Design review of the part built by this model. Coordinates are the model's own, in mm. A direction names the side the tool comes from. Give positions to 0.01 mm unless a question says otherwise; leave off trailing zeros. Loops run counter-clockwise (first coordinate to the right, second up) from the corner with the lowest first, then second, coordinate; pieces in that order, holes last. Notation, with made-up numbers: M 84.5,15.25 L 120.5,15.25 A13 ccw 120.5,35.25 Z; hole C 51,34.5 d3. An arc over 180 degrees is marked long. Use a Markdown table: item, result. Add a question column.
(1) Draft analysis for pull direction X (two halves, no side actions). For faces 3 (the face through (-427, 7, -650)), 4 (the face through (-311.84, 8.526, -537.131)), 5 (the face through (-650, 7, -427)), 6 (the face through (-536.16, 8.526, -310.869)), state which applies: pulls with the +X half, pulls with the -X half, needs draft (parallel to the pull), parting line crosses it, or undercut.
(2) For faces 1 (the face through (-536.16, 8.526, -537.131)), 2 (the face through (-427, 14.5, -421)), list the 3-axis set-ups (+Z, -Z, +X, -X, +Y, -Y) from which the entire face can be reached by the end or side of a thin tool; tool diameter is ignored.
(3) Add section A-A, the plane x = -546. Give the boundary of the cut face in (y, z) (3 decimals), then the cut area to 3 significant figures.
(4) Insertion check: pin 1 Ø3.5 at (x, z) = (-281, -326) entering from -Y. The pin has a flat end and moves straight along its axis. Give the tip position at first contact, or say it passes through.
(5) For probe 1 along X at (y, z) = (9, -552); probe 2 along Z at (x, y) = (-567, 6); probe 3 along Z at (x, y) = (-515, 9), list the stretches that pass through material, from the lowest coordinate up.
```python
from build123d import *

# Parameters (mm, degrees)
SKETCH1_W               = 452
SKETCH1_H               = 452
BOSS_EXTRUDE1_DEPTH     = 15
SKETCH15_R              = 5.975
CUT_EXTRUDE12_DEPTH     = 120
MIRROR2_COPY_1_SKETCH_R = 5.975
MIRROR2_COPY_1_DEPTH    = 120
SKETCH16_R              = 3
CUT_EXTRUDE13_DEPTH     = 120
SKETCH17_R              = 4.1
SKETCH17_R_2            = 4.25
CUT_EXTRUDE14_DEPTH     = 120
MIRROR4_COPY_1_SKETCH_R = 3
MIRROR4_COPY_1_DEPTH    = 120


with BuildPart() as part:
    # Sketch1 → Boss-Extrude1 (new body)
    with BuildSketch(Plane.XZ.offset(0.5)):
        with Locations((-424, -424)):
            Rectangle(SKETCH1_W, SKETCH1_H)
    extrude(amount=-BOSS_EXTRUDE1_DEPTH)

    # Sketch15 → Cut-Extrude12 (cut)
    with BuildSketch(Plane(origin=(-477, 324.820623632, -300), x_dir=(0, 0, 1), z_dir=(1, 0, 0))):
        with Locations((-11, 310.320623632)):
            Circle(SKETCH15_R)
    cut_extrude12 = extrude(amount=-CUT_EXTRUDE12_DEPTH, mode=Mode.SUBTRACT)

    # Mirror1: Cut-Extrude12 across plane
    add(cut_extrude12.mirror(Plane(origin=(0, 0, -424), x_dir=(1, 0, 0), z_dir=(0, 0, -1))), mode=Mode.SUBTRACT)

    # Mirror2: Cut-Extrude12 across plane
    add(cut_extrude12.mirror(Plane.ZY.offset(424)), mode=Mode.SUBTRACT)

    # Mirror2 copy 1 sketch → Mirror2 copy 1 (cut)
    with BuildSketch(Plane(origin=(-371, 324.820623632, -548), x_dir=(0, 0, -1), z_dir=(-1, 0, 0))):
        with Locations((-11, 310.320623632)):
            Circle(MIRROR2_COPY_1_SKETCH_R)
    extrude(amount=-MIRROR2_COPY_1_DEPTH, mode=Mode.SUBTRACT)

    # Sketch16 → Cut-Extrude13 (cut)
    with BuildSketch(Plane(origin=(-300, 101.5, -300), x_dir=(-1, 0, 0), z_dir=(0, 1, 0))):
        with Locations(Location((-19, -26, 0), (0, 0, 270))):
            Circle(SKETCH16_R)
        with Locations(Location((41, -26, 0), (0, 0, 270))):
            Circle(SKETCH16_R)
        with Locations(Location((41, 4, 0), (0, 0, 270))):
            Circle(SKETCH16_R)
        with Locations(Location((-19, 4, 0), (0, 0, 270))):
            Circle(SKETCH16_R)
    cut_extrude13 = extrude(amount=-CUT_EXTRUDE13_DEPTH, mode=Mode.SUBTRACT)

    # Sketch17 → Cut-Extrude14 (cut)
    with BuildSketch(Plane(origin=(-300, 101.5, -300), x_dir=(-1, 0, 0), z_dir=(0, 1, 0))):
        with Locations(Location((327.071067812, -326.871067812, 0), (0, 0, 270))):
            Circle(SKETCH17_R)
        with Locations(Location((-79.071067812, -326.871067812, 0), (0, 0, 270))):
            Circle(SKETCH17_R)
        with Locations(Location((103.571067812, -144.328932188, 0), (0, 0, 270))):
            Circle(SKETCH17_R_2)
        with Locations(Location((327.071067812, 79.071067812, 0), (0, 0, 270))):
            Circle(SKETCH17_R)
        with Locations(Location((-79.071067812, 79.071067812, 0), (0, 0, 270))):
            Circle(SKETCH17_R)
    extrude(amount=-CUT_EXTRUDE14_DEPTH, mode=Mode.SUBTRACT)

    # Mirror3: Cut-Extrude13 across plane
    add(cut_extrude13.mirror(Plane.ZY.offset(424)), mode=Mode.SUBTRACT)

    # Mirror4: Cut-Extrude13 across plane
    add(cut_extrude13.mirror(Plane(origin=(0, 0, -424), x_dir=(1, 0, 0), z_dir=(0, 0, -1))), mode=Mode.SUBTRACT)

    # Mirror4 copy 1 sketch → Mirror4 copy 1 (cut)
    with BuildSketch(Plane(origin=(-548, 101.5, -548), x_dir=(1, 0, 0), z_dir=(0, 1, 0))):
        with Locations(Location((-19, -26, 0), (0, 0, 270))):
            Circle(MIRROR4_COPY_1_SKETCH_R)
        with Locations(Location((41, -26, 0), (0, 0, 270))):
            Circle(MIRROR4_COPY_1_SKETCH_R)
        with Locations(Location((41, 4, 0), (0, 0, 270))):
            Circle(MIRROR4_COPY_1_SKETCH_R)
        with Locations(Location((-19, 4, 0), (0, 0, 270))):
            Circle(MIRROR4_COPY_1_SKETCH_R)
    extrude(amount=-MIRROR4_COPY_1_DEPTH, mode=Mode.SUBTRACT)


solid = part.part
```
Established:
| question | item | result |
|---|---|---|
| 1 | face 3 | needs draft |
| 1 | face 4 | undercut |
| 1 | face 5 | pulls with the -X half |
| 1 | face 6 | undercut |
| 2 | face 1 | +Y |
| 2 | face 2 | +Z, -Z, +X, -X, +Y |
| 3 | outline | M -0.5,-650 L 14.5,-650 L 14.5,-542.975 A5.975 cw 14.5,-531.025 L 14.5,-316.975 A5.975 cw 14.5,-305.025 L 14.5,-198 L -0.5,-198 Z |
| 3 | area | 6,670 mm^2 |
| 4 | pin 1 | through |
| 5 | probe 1 | -650 to -570, -564 to -510, -504 to -344, -338 to -284, -278 to -198 |
| 5 | probe 2 | -650 to -555, -549 to -525, -519 to -329, -323 to -299, -293 to -198 |
| 5 | probe 3 | -650 to -539.33, -534.67 to -313.33, -308.67 to -198 |
